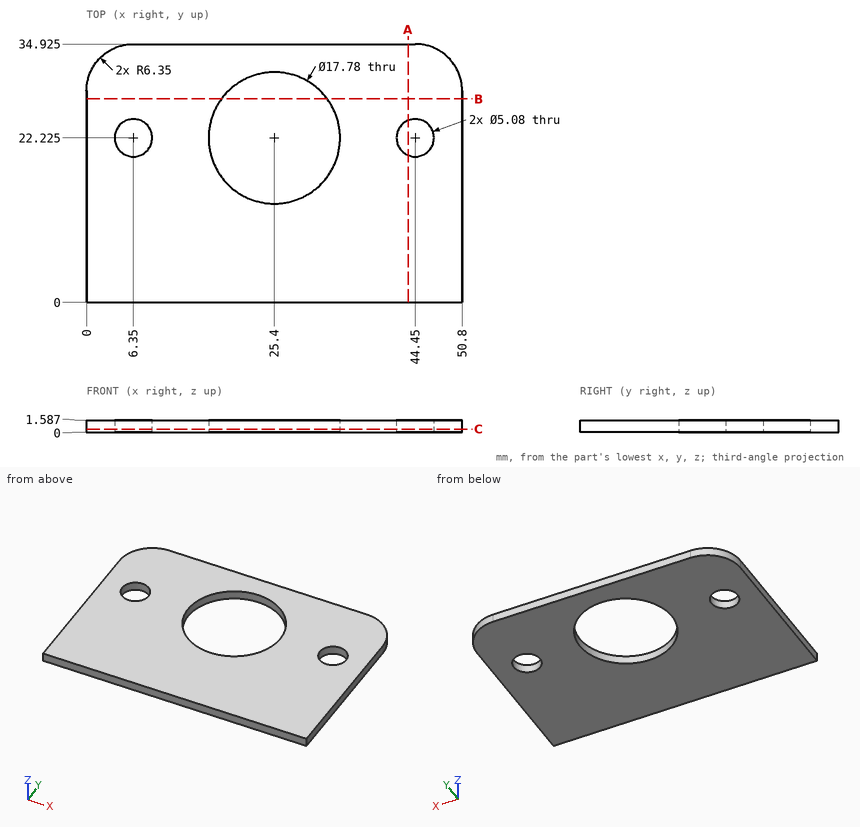
Source: three-view drawing plus pictorial views. Frame: mm from the lowest corner of the part. Give positions to 0.01 mm unless a question says otherwise; leave off trailing zeros. Order: outer loops, then holes, each group sorted by start corner. A loop starts at its lowest first (then second) coordinate and runs counter-clockwise, first axis right, second up. Notation, with made-up numbers: (8, -22) - (51, -22) arc R4 ccw to (51, -18) - close; hole circle Ø1 at (68.25, -21.75). An arc over 180 degrees is marked (long way). Answer as a JSON object with one key per item and string values. Group by question number.
Q1. Line query: probe 1 along X at (y, z) = (24, 1.2) (1 decimal); probe 2 along Y at (x, z) = (6.35, 0.95) (1 decimal); probe 3 along Y at (x, z) = (20, 1.2) (1 decimal). Output: solid intervals per line, ascending.
Q2. Cut plane A-A, the plane x = 43.5. Output: boundary loops of the cut face in (y, z) (1 decimal).
Q3. Cut plane B-B, the plane y = 27.5. Output: boundary loops of the cut face in (x, z) (1 decimal).
Q4. Cut plane C-C, the plane z = 0.4. Count the separate pieces of the cut face and the enclosed holes in it, then the cut area to 3 significant figures.
Results:
{
 "1": {"probe 1": "0 to 4.5, 8.2 to 16.7, 34.1 to 42.6, 46.3 to 50.8", "probe 2": "0 to 19.7, 24.8 to 34.9", "probe 3": "0 to 15.2, 29.3 to 34.9"},
 "2": {"outline": "(0, 0) - (19.9, 0) - (19.9, 1.6) - (0, 1.6) - close; (24.6, 0) - (34.9, 0) - (34.9, 1.6) - (24.6, 1.6) - close"},
 "3": {"outline": "(0, 0) - (18.2, 0) - (18.2, 1.6) - (0, 1.6) - close; (32.6, 0) - (50.8, 0) - (50.8, 1.6) - (32.6, 1.6) - close"},
 "4": {"separate pieces": "1", "enclosed holes": "3", "area": "1,470 mm^2"}
}
